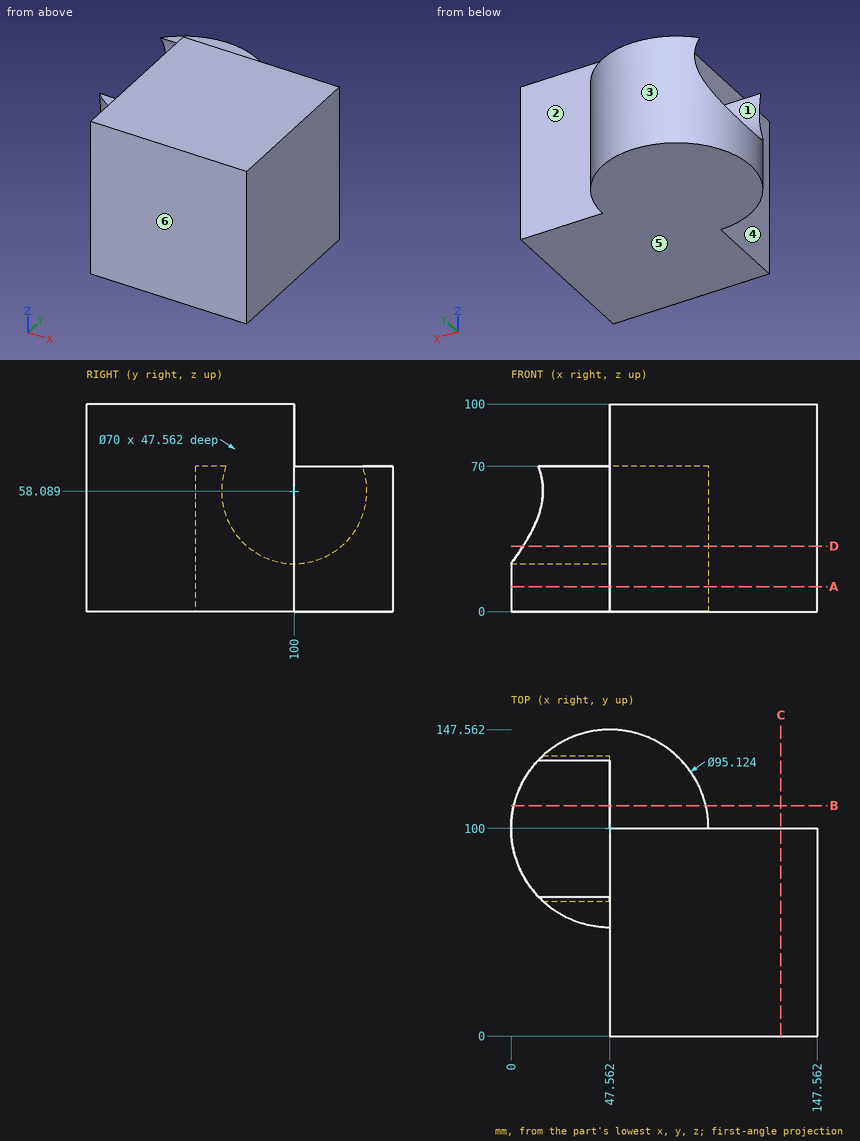
Geometry: see drawing. Coordinates: mm, zero at the bounding-box minimum. A direction names the side the tool comes from. Coordinates: 2 decimals unless noted, no trailing zeros. Loops run counter-clockwise (first coordinate to the right, second up) from the corner with the lowest first, then second, coordinate; pieces in that order, holes last. Notation, with made-up numbers: (46, -0.75) - (51, -0.75) arc R25 ccw to (51, 24.25) - close; hole circle Ø8 at (40.25, 24). An arc over 180 degrees is marked (long way). Put each result on its own line as item: value. Start each with the question number.
Q1. Pin query (flat end, axial travel): pin 1 Ø11.5 at (x, y) = (28.5, 62.5) entering from +Z; pin 2 Ø10 at (x, y) = (32, 87.5) entering from +Z. Return the tip coordinate at first contact, or that it passes through.
Q2. Cut plane B-B, the plane y = 111. Return loops of the section in (x, z) (1 decimal), and give its area (3 significant figures).
Q3. Set-up query: the marked faces 1, 2 and 3. Return all of +Z, -Z, +X, -X, +Y, -Y with unobstructed straight access to the full face (end or side cutting, diameter ignored); none if empty.
Q4. Cut plane A-A, the plane z = 12. Return loops of the section in (x, y).
Q5. Line query: line 1 (Y direction, x = 54, z = 80); line 2 (Z direction, x = 29, y = 100); line 3 (X direction, y = 18, z = 13). Output: solid intervals per line, ascending.
Q6. Pull-direction query (Y, two-part tool) for the marked faces 4, 5 and 6; classes: released by +Y, released by -Y, zero draft, split by the parting line, or undercut.
Q7. Cut plane D-D, the plane z = 31.5. Return loops of the section in (x, y), and give its area (3 significant figures).
Q8. Cut plane C-C, the plane x = 130. Return loops of the section in (y, z), and give its area (3 significant figures).
Filled sheet:
1. pin 1: z = 70
1. pin 2: z = 27.78
2. outline: (1.3, 0) - (93.8, 0) - (93.8, 70) - (47.6, 70) - (47.6, 24.9) - (1.3, 24.9) - close
2. area: 4,390 mm²
3. face 1: -X
3. face 2: +Z, +X, +Y
3. face 3: +Z, -Z
4. outline: (47.56, 0) - (147.56, 0) - (147.56, 100) - (95.12, 100) arc R47.56 ccw (long way) to (47.56, 52.44) - close
5. line 1: 0 to 100
5. line 2: 0 to 23.09
5. line 3: 47.56 to 147.56
6. face 4: undercut
6. face 5: zero draft
6. face 6: released by -Y
7. outline: (5.8, 77.24) arc R47.56 ccw to (47.56, 52.44) - (47.56, 0) - (147.56, 0) - (147.56, 100) - (95.12, 100) arc R47.56 ccw to (5.8, 122.76) - (47.56, 122.76) - (47.56, 77.24) - close
7. area: 13,300 mm²
8. outline: (0, 0) - (100, 0) - (100, 100) - (0, 100) - close
8. area: 10,000 mm²
